Verification items for the finished model (mm, model axes). Give positions to 0.01 mm unless a question says otherwise; leave off trailing zeros. Order: outer loops, then holes, each group sorted by start corner. A loop starts at its lowest first (then second) coordinate and runs counter-clockwise, first axis right, second up. Notation, with made-up numbers: (52.5, 52.5) -> (100.5, 52.5) arc R27 cw to (100.5, 80.5) -> close; hole circle Ø3 at (-16, -9.75). An arc over 180 degrees is marked (long way). Return JSON: item names as keys, results as strings. Group by question number.
(1) Cross-section at B-B on z = 1.95. State how many separate pieces and enclosed holes the cut face has, then the cut area to 3 significant figures.
(2) Thickness scan on line 1 along Y through (x, z) = (-103.5, 2.9); line 2 along X through (y, z) = (330, 2.6); line 3 along Y through (x, z) = (-64, 0.5). Record the ranges inside material, lowest first.
(3) Cross-section at A-A on y = 268. Enter the section's corners in (x, z), then the cut area to 3 significant figures.
(4) Depth check by flat-ended pin: pin 1 Ø1.5 at (x, z) = (-27.5, 3.5) entering from -Y; pin 2 Ø1.5 at (x, z) = (-104, 3) entering from -Y; pin 3 Ø1.5 at (x, z) = (-35.5, 2.5) entering from +Y; pin 4 Ø5.5 at (x, y) = (-103.5, 287.5) entering from +Z. Enter the tip coordinate at first touch or a pass-through.
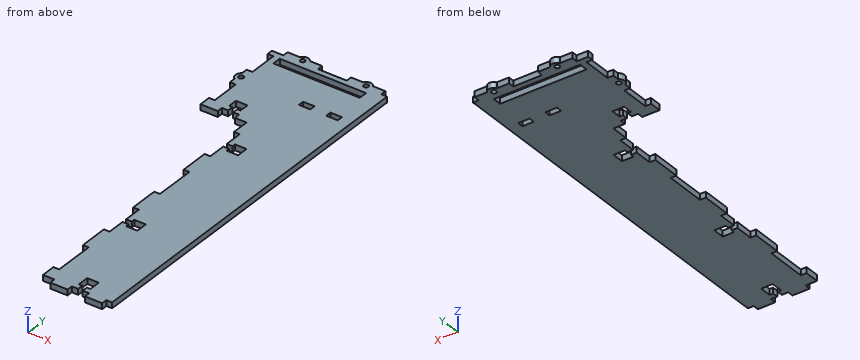
from build123d import *

# Parameters (mm, degrees)
SKETCH1_W           = 106
SKETCH1_H           = 327.5
BOSS_EXTRUDE1_DEPTH = 5
SKETCH2_W           = 40
SKETCH2_H           = 242.5
CUT_EXTRUDE1_DEPTH  = 5
SKETCH3_W           = 5
SKETCH3_H           = 25
CUT_EXTRUDE2_DEPTH  = 5
SKETCH4_W           = 30
SKETCH4_H           = 5
BOSS_EXTRUDE2_DEPTH = 5
SKETCH5_W           = 15
SKETCH5_H           = 5
CUT_EXTRUDE3_DEPTH  = 5
SKETCH6_W           = 5
SKETCH6_H           = 35
CUT_EXTRUDE4_DEPTH  = 5
SKETCH7_W           = 10
SKETCH7_H           = 5
CUT_EXTRUDE5_DEPTH  = 5
SKETCH8_W           = 15
SKETCH8_H           = 5
BOSS_EXTRUDE3_DEPTH = 5
SKETCH9_W           = 70
SKETCH9_H           = 7.5
CUT_EXTRUDE6_DEPTH  = 5
SKETCH10_W          = 5
SKETCH10_H          = 227.5
BOSS_EXTRUDE4_DEPTH = 5
SKETCH11_R          = 2.1
CUT_EXTRUDE7_DEPTH  = 5
BOSS_EXTRUDE5_DEPTH = 5
SKETCH13_W          = 10
SKETCH13_H          = 327.5
SKETCH13_W_2        = 11.118393302
SKETCH13_H_2        = 31.265749724
SKETCH13_W_3        = 24.993123917
SKETCH13_H_3        = 36.030112223
CUT_EXTRUDE8_DEPTH  = 10
SKETCH14_W          = 5
SKETCH14_H          = 327.5
CUT_EXTRUDE9_DEPTH  = 1
SKETCH15_W          = 4.2
SKETCH15_H          = 5
SKETCH15_W_2        = 5
SKETCH15_H_2        = 4.2
SKETCH15_W_3        = 10
SKETCH15_H_3        = 10
CUT_EXTRUDE10_DEPTH = 10
SKETCH16_R          = 2.1
CUT_EXTRUDE11_DEPTH = 10
BOSS_EXTRUDE6_DEPTH = 5
SKETCH19_W          = 4
SKETCH19_H          = 5
CUT_EXTRUDE13_DEPTH = 5
SKETCH20_R          = 2.1
CUT_EXTRUDE14_DEPTH = 5
BOSS_EXTRUDE7_DEPTH = 5
SKETCH22_W          = 5
SKETCH22_H          = 7.5
CUT_EXTRUDE15_DEPTH = 5


with BuildPart() as part:
    # Sketch1 → Boss-Extrude1 (new body)
    with BuildSketch(Plane.XY):
        with Locations((-53, 163.75)):
            Rectangle(SKETCH1_W, SKETCH1_H)
    extrude(amount=BOSS_EXTRUDE1_DEPTH)

    # Sketch2 → Cut-Extrude1 (cut)
    with BuildSketch(Plane.XY.offset(5)):
        with Locations((-86, 121.25)):
            Rectangle(SKETCH2_W, SKETCH2_H)
    extrude(amount=-CUT_EXTRUDE1_DEPTH, mode=Mode.SUBTRACT)

    # Sketch3 → Cut-Extrude2 (cut)
    with BuildSketch(Plane.XY.offset(5)):
        with Locations((-103.5, 310)):
            Rectangle(SKETCH3_W, SKETCH3_H)
        with Locations((-103.5, 265)):
            Rectangle(SKETCH3_W, SKETCH3_H)
    extrude(amount=-CUT_EXTRUDE2_DEPTH, mode=Mode.SUBTRACT)

    # Sketch4 → Boss-Extrude2 (add)
    with BuildSketch(Plane.XY.offset(5)):
        with Locations((-26, 330)):
            Rectangle(SKETCH4_W, SKETCH4_H)
        with Locations((-81, 330)):
            Rectangle(SKETCH4_W, SKETCH4_H)
    extrude(amount=-BOSS_EXTRUDE2_DEPTH)

    # Sketch5 → Cut-Extrude3 (cut)
    with BuildSketch(Plane.XY.offset(5)):
        with Locations((-83.5, 245)):
            Rectangle(SKETCH5_W, SKETCH5_H)
    extrude(amount=-CUT_EXTRUDE3_DEPTH, mode=Mode.SUBTRACT)

    # Sketch6 → Cut-Extrude4 (cut)
    with BuildSketch(Plane.XY.offset(5)):
        with Locations((-63.5, 210)):
            Rectangle(SKETCH6_W, SKETCH6_H)
        with Locations((-63.5, 150)):
            Rectangle(SKETCH6_W, SKETCH6_H)
        with Locations((-63.5, 90)):
            Rectangle(SKETCH6_W, SKETCH6_H)
        with Locations((-63.5, 30)):
            Rectangle(SKETCH6_W, SKETCH6_H)
    extrude(amount=-CUT_EXTRUDE4_DEPTH, mode=Mode.SUBTRACT)

    # Sketch7 → Cut-Extrude5 (cut)
    with BuildSketch(Plane.XY.offset(5)):
        with Locations((-21, 285)):
            Rectangle(SKETCH7_W, SKETCH7_H)
        with Locations((-44.75, 285)):
            Rectangle(SKETCH7_W, SKETCH7_H)
    extrude(amount=-CUT_EXTRUDE5_DEPTH, mode=Mode.SUBTRACT)

    # Sketch8 → Boss-Extrude3 (add)
    with BuildSketch(Plane.XY.offset(5)):
        with Locations((-18.5, -2.5)):
            Rectangle(SKETCH8_W, SKETCH8_H)
        with Locations((-48.5, -2.5)):
            Rectangle(SKETCH8_W, SKETCH8_H)
    extrude(amount=-BOSS_EXTRUDE3_DEPTH)

    # Sketch9 → Cut-Extrude6 (cut)
    with BuildSketch(Plane(origin=(0, 0, 0), x_dir=(-1, 0, 0), z_dir=(0, 0, -1))):
        with Locations((55.5, 318.75)):
            Rectangle(SKETCH9_W, SKETCH9_H)
    extrude(amount=-CUT_EXTRUDE6_DEPTH, mode=Mode.SUBTRACT)

    # Sketch10 → Boss-Extrude4 (add)
    with BuildSketch(Plane(origin=(0, 0, 0), x_dir=(-1, 0, 0), z_dir=(0, 0, -1))):
        with Locations((-2.5, 163.75)):
            Rectangle(SKETCH10_W, SKETCH10_H)
    extrude(amount=-BOSS_EXTRUDE4_DEPTH)

    # Sketch11 → Cut-Extrude7 (cut)
    with BuildSketch(Plane(origin=(0, 0, 0), x_dir=(-1, 0, 0), z_dir=(0, 0, -1))):
        with Locations((-2.5, 75)):
            Circle(SKETCH11_R)
        with Locations((-2.5, 252.5)):
            Circle(SKETCH11_R)
    extrude(amount=-CUT_EXTRUDE7_DEPTH, mode=Mode.SUBTRACT)

    # Sketch12 → Boss-Extrude5 (add)
    with BuildSketch(Plane(origin=(0, 0, 0), x_dir=(-1, 0, 0), z_dir=(0, 0, -1))):
        with BuildLine():
            Line((-5, 70.669872981), (-5, 79.330127019))
            ThreePointArc((-5, 79.330127019), (-7.5, 75), (-5, 70.669872981))
        make_face()
        with BuildLine():
            Line((-5, 256.830127019), (-5, 248.169872981))
            ThreePointArc((-5, 248.169872981), (-7.5, 252.5), (-5, 256.830127019))
        make_face()
    extrude(amount=-BOSS_EXTRUDE5_DEPTH)

    # Sketch13 → Cut-Extrude8 (cut)
    with BuildSketch(Plane(origin=(0, 0, 0), x_dir=(-1, 0, 0), z_dir=(0, 0, -1))):
        with Locations((0, 163.75)):
            Rectangle(SKETCH13_W, SKETCH13_H)
        with Locations((-10.559196651, 252.176794505)):
            Rectangle(SKETCH13_W_2, SKETCH13_H_2)
        with Locations((-17.496561959, 79.007982861)):
            Rectangle(SKETCH13_W_3, SKETCH13_H_3)
    extrude(amount=-CUT_EXTRUDE8_DEPTH, mode=Mode.SUBTRACT)

    # Sketch14 → Cut-Extrude9 (cut)
    with BuildSketch(Plane(origin=(-5, 0, 0), x_dir=(0, 0, -1), z_dir=(1, 0, 0))):
        with Locations((-2.5, 163.75)):
            Rectangle(SKETCH14_W, SKETCH14_H)
    extrude(amount=-CUT_EXTRUDE9_DEPTH, mode=Mode.SUBTRACT)

    # Sketch15 → Cut-Extrude10 (cut)
    with BuildSketch(Plane(origin=(0, 0, 0), x_dir=(-1, 0, 0), z_dir=(0, 0, -1))):
        Polygon((78.5, 252.5), (81.4, 252.5), (85.6, 252.5), (88.5, 252.5), (88.5, 260.7), (78.5, 260.7), align=None)
        with Locations((83.5, 250)):
            Rectangle(SKETCH15_W, SKETCH15_H)
        Polygon((56, 207.9), (56, 212.1), (56, 215), (46, 215), (46, 205), (56, 205), align=None)
        with Locations((58.5, 210)):
            Rectangle(SKETCH15_W_2, SKETCH15_H_2)
        with Locations((51, 90)):
            Rectangle(SKETCH15_W_3, SKETCH15_H_3)
        with Locations((58.5, 90)):
            Rectangle(SKETCH15_W_2, SKETCH15_H_2)
    extrude(amount=-CUT_EXTRUDE10_DEPTH, mode=Mode.SUBTRACT)

    # Sketch16 → Cut-Extrude11 (cut)
    with BuildSketch(Plane(origin=(0, 0, 0), x_dir=(-1, 0, 0), z_dir=(0, 0, -1))):
        with Locations((103.5, 287.5)):
            Circle(SKETCH16_R)
    extrude(amount=-CUT_EXTRUDE11_DEPTH, mode=Mode.SUBTRACT)

    # Sketch17 → Boss-Extrude6 (add)
    with BuildSketch(Plane(origin=(0, 0, 0), x_dir=(-1, 0, 0), z_dir=(0, 0, -1))):
        with BuildLine():
            Line((106, 283.169872981), (106, 291.830127019))
            ThreePointArc((106, 291.830127019), (108.5, 287.5), (106, 283.169872981))
        make_face()
    extrude(amount=-BOSS_EXTRUDE6_DEPTH)

    # Sketch19 → Cut-Extrude13 (cut)
    with BuildSketch(Plane.XY.offset(5)):
        with Locations((-33.5, 2.5)):
            Rectangle(SKETCH19_W, SKETCH19_H)
        Polygon((-38.5, 5), (-35.5, 5), (-31.5, 5), (-28.5, 5), (-28.5, 15), (-38.5, 15), align=None)
    extrude(amount=-CUT_EXTRUDE13_DEPTH, mode=Mode.SUBTRACT)

    # Sketch20 → Cut-Extrude14 (cut)
    with BuildSketch(Plane(origin=(0, 0, 0), x_dir=(-1, 0, 0), z_dir=(0, 0, -1))):
        with Locations((26, 330)):
            Circle(SKETCH20_R)
        with Locations((81, 330)):
            Circle(SKETCH20_R)
    extrude(amount=-CUT_EXTRUDE14_DEPTH, mode=Mode.SUBTRACT)

    # Sketch21 → Boss-Extrude7 (add)
    with BuildSketch(Plane(origin=(0, 0, 0), x_dir=(-1, 0, 0), z_dir=(0, 0, -1))):
        with BuildLine():
            Line((30.330127019, 332.5), (21.669872981, 332.5))
            ThreePointArc((21.669872981, 332.5), (26, 335), (30.330127019, 332.5))
        make_face()
        with BuildLine():
            Line((76.669872981, 332.5), (85.330127019, 332.5))
            ThreePointArc((85.330127019, 332.5), (81, 335), (76.669872981, 332.5))
        make_face()
    extrude(amount=-BOSS_EXTRUDE7_DEPTH)

    # Sketch22 → Cut-Extrude15 (cut)
    with BuildSketch(Plane(origin=(0, 0, 0), x_dir=(-1, 0, 0), z_dir=(0, 0, -1))):
        with Locations((93, 318.75)):
            Rectangle(SKETCH22_W, SKETCH22_H)
    extrude(amount=-CUT_EXTRUDE15_DEPTH, mode=Mode.SUBTRACT)


solid = part.part
Verdict:
{
 "1": {"separate pieces": "1", "enclosed holes": "6", "area": "21,400 mm²"},
 "2": {"line 1": "242.5 to 252.5, 277.5 to 285.4, 289.6 to 297.5, 322.5 to 327.5", "line 2": "-96 to -83.1, -78.9 to -66, -41 to -28.1, -23.9 to -11", "line 3": "0 to 12.5, 47.5 to 72.5, 107.5 to 132.5, 167.5 to 192.5, 227.5 to 315, 322.5 to 327.5"},
 "3": {"outline": "(-101, 0) -> (-6, 0) -> (-6, 5) -> (-101, 5) -> close", "area": "475 mm²"},
 "4": {"pin 1": "y = 0", "pin 2": "y = 242.5", "pin 3": "y = 332.5", "pin 4": "z = 5"}
}
